The model under review builds one solid part; all positions refer to its coordinate system, in mm. Face numbers are marked on the shaded views. A direction names the side the tool comes from. Give positions to 0.01 mm unless a question says otherwise; leave off trailing zeros. Order: outer loops, then holes, each group sorted by start corner. A loop starts at its lowest first (then second) coordinate and runs counter-clockwise, first axis right, second up. Notation, with made-up numbers: (64.5, 24) - (105.5, 24) arc R26 ccw to (105.5, 45) - close; hole circle Ø5 at (23.5, 82.25). An arc over 180 degrees is marked (long way). Use CSV: the item, a comma, the result in double quotes. Start each with the question number.
1. To check wall thickness, follow line 1 (Y direction, x = -3, z = 34.5); line 2 (X direction, y = -121.5, z = 29.5); line 3 (Y direction, x = -38, z = 80.5). State the ranges of each line that lie inside material, in increasing order. Write a range as [from, to].
2. For pin 1 (2 mm diameter, centred on x = 18.5, y = 36, fed in from -Z); pin 2 (4 mm diameter, centred on x = -38.5, z = -49, fed in from +Y); pin 3 (5 mm diameter, centred on x = -0.5, z = 26.5, fed in from +Y), all flat-tipped, find the tip position at first contact; note any pin that passes through.
3. Take a section at D-D, the plane x = -55. State the section outline as (y, z) points, then the cut area to 3 significant figures.
4. Take a section at A-A, the plane z = 110. State the section outline as (x, y) points.
5. Take a section at B-B, the plane z = 83.5. State the section outline as (x, y) points.
6. Take a section at C-C, the plane y = -54.5. State the section outline as (x, z) points, then the cut area to 3 significant figures.
7. Machinability: for the marked faces 1, 2 and 3, which of the approach directions +Z, -Z, +X, -X, +Y, -Y give a long, thin tool a straight path to every point of the face, cutting with its end or side? Answer none if there is none.
8. Draft analysis for pull direction Y (two halves, no side actions). For the marked faces 4, 5 and 6, state which applies: released by +Y, released by -Y, zero draft, split by the parting line, or undercut.
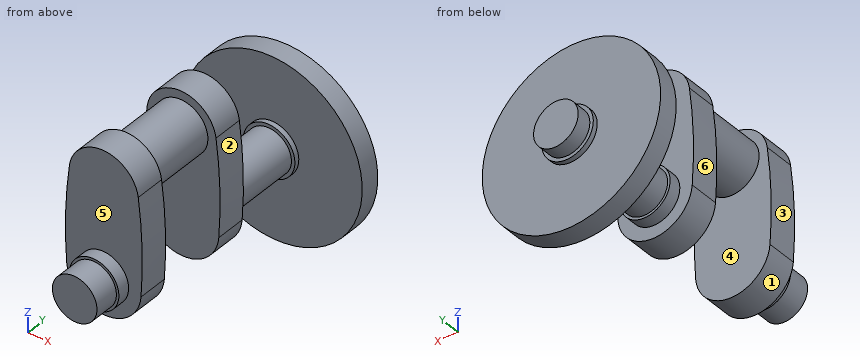
```python
from build123d import *

# Parameters (mm, degrees)
SKETCH1_R           = 22.5
BOSS_EXTRUDE1_DEPTH = 25
SKETCH2_R           = 25
BOSS_EXTRUDE2_DEPTH = 12.5
BOSS_EXTRUDE3_DEPTH = 30
SKETCH4_R           = 26.5
BOSS_EXTRUDE4_DEPTH = 35
SKETCH5_R           = 22.5
BOSS_EXTRUDE5_DEPTH = 50
SKETCH6_R           = 90
BOSS_EXTRUDE6_DEPTH = 20
SKETCH7_R           = 22.5
BOSS_EXTRUDE7_DEPTH = 20
SKETCH8_R           = 26
BOSS_EXTRUDE8_DEPTH = 5
BOSS_EXTRUDE9_START = 5
SKETCH9_R           = 26
BOSS_EXTRUDE9_DEPTH = 5


with BuildPart() as part:
    # Sketch1 → Boss-Extrude1 (new body)
    with BuildSketch(Plane(origin=(0, 0, 0), x_dir=(1, 0, 0), z_dir=(0, 1, 0))):
        with Locations(Location((0, 0, 0), (0, 0, 270))):
            Circle(SKETCH1_R)
    extrude(amount=BOSS_EXTRUDE1_DEPTH)

    # Sketch2 → Boss-Extrude2 (add)
    with BuildSketch(Plane(origin=(0, 0, 0), x_dir=(1, 0, 0), z_dir=(0, 1, 0))):
        with Locations(Location((0, 0, 0), (0, 0, 270))):
            Circle(SKETCH2_R)
    extrude(amount=-BOSS_EXTRUDE2_DEPTH)

    # Sketch3 → Boss-Extrude3 (add)
    with BuildSketch(Plane.XZ.offset(12.5)):
        with BuildLine():
            ThreePointArc((-37.5, -2.740437921), (0, -37.6), (37.5, -2.740437921))
            ThreePointArc((37.5, -2.740437921), (38.576956863, 45.97711937), (34.702685351, 94.552321322))
            ThreePointArc((34.702685351, 94.552321322), (0, 125), (-34.702685351, 94.552321322))
            ThreePointArc((-34.702685351, 94.552321322), (-38.576956863, 45.97711937), (-37.5, -2.740437921))
        make_face()
    extrude(amount=BOSS_EXTRUDE3_DEPTH)

    # Sketch4 → Boss-Extrude4 (add)
    with BuildSketch(Plane.XZ.offset(42.5)):
        with Locations(Location((0, 90, 0), (0, 0, 270))):
            Circle(SKETCH4_R)
    extrude(amount=BOSS_EXTRUDE4_DEPTH)

    # Mirror1: part across plane


with BuildPart() as part_1:
    add(part.part)
    add(part.part.mirror(Plane(origin=(0, -77.5, 90), x_dir=(0, 0, 1), z_dir=(0, -1, 0))))

    # Sketch5 → Boss-Extrude5 (add)
    with BuildSketch(Plane(origin=(0, 25, 0), x_dir=(1, 0, 0), z_dir=(0, 1, 0))):
        with Locations(Location((0, 0, 0), (0, 0, 270))):
            Circle(SKETCH5_R)
    extrude(amount=BOSS_EXTRUDE5_DEPTH)

    # Sketch6 → Boss-Extrude6 (add)
    with BuildSketch(Plane(origin=(0, 75, 0), x_dir=(1, 0, 0), z_dir=(0, 1, 0))):
        with Locations(Location((0, 0, 0), (0, 0, 270))):
            Circle(SKETCH6_R)
    extrude(amount=BOSS_EXTRUDE6_DEPTH)

    # Sketch7 → Boss-Extrude7 (add)
    with BuildSketch(Plane(origin=(0, 95, 0), x_dir=(1, 0, 0), z_dir=(0, 1, 0))):
        with Locations(Location((0, 0, 0), (0, 0, 270))):
            Circle(SKETCH7_R)
    extrude(amount=BOSS_EXTRUDE7_DEPTH)

    # Sketch8 → Boss-Extrude8 (add)
    with BuildSketch(Plane.XZ.offset(-75)):
        with Locations(Location((0, 0, 0), (0, 0, 90))):
            Circle(SKETCH8_R)
    extrude(amount=BOSS_EXTRUDE8_DEPTH)

    # Sketch9 → Boss-Extrude9 (add)
    with BuildSketch(Plane(origin=(0, 95, 0), x_dir=(1, 0, 0), z_dir=(0, 1, 0)).offset(BOSS_EXTRUDE9_START)):
        with Locations(Location((0, 0, 0), (0, 0, 270))):
            Circle(SKETCH9_R)
    extrude(amount=-BOSS_EXTRUDE9_DEPTH)


solid = part_1.part
```
Determined:
1,line 1,"y = [-142.5, -112.5], [-42.5, -12.5], [75, 95]"
1,line 2,"x = [-38.77, 38.77]"
1,line 3,"y = [75, 95]"
2,pin 1,"stops at z = -14.14"
2,pin 2,"stops at y = 95"
2,pin 3,"stops at y = 100"
3,outline,"(75, -71.24) - (95, -71.24) - (95, 71.24) - (75, 71.24) - close"
3,area,"2,850 mm²"
4,outline,"(-28.72, -142.5) - (28.72, -142.5) - (28.72, -112.5) - (17.39, -112.5) - (17.39, -42.5) - (28.72, -42.5) - (28.72, -12.5) - (-28.72, -12.5) - (-28.72, -42.5) - (-17.39, -42.5) - (-17.39, -112.5) - (-28.72, -112.5) - close"
5,outline,"(-36.02, -142.5) - (36.02, -142.5) - (36.02, -112.5) - (25.69, -112.5) - (25.69, -42.5) - (36.02, -42.5) - (36.02, -12.5) - (-36.02, -12.5) - (-36.02, -42.5) - (-25.69, -42.5) - (-25.69, -112.5) - (-36.02, -112.5) - close; (-33.58, 75) - (33.58, 75) - (33.58, 95) - (-33.58, 95) - close"
6,outline,"circle Ø53 at (0, 90)"
6,area,"2,210 mm²"
7,face 1,"-Z, -Y"
7,face 2,"+X, -Y"
7,face 3,"-X, -Y"
8,face 4,"undercut"
8,face 5,"released by -Y"
8,face 6,"zero draft"
